```python
from build123d import *

# Parameters (mm, degrees)
SKETCH1_R           = 16.5
BOSS_EXTRUDE1_DEPTH = 82
SKETCH2_R           = 11
CUT_EXTRUDE1_DEPTH  = 276.268959383
SKETCH5_W           = 65
SKETCH5_H           = 35
CUT_EXTRUDE2_DEPTH  = 282.890049487
CUT_EXTRUDE3_DEPTH  = 40


with BuildPart() as part:
    # Sketch1 → Boss-Extrude1 (new body)
    with BuildSketch(Plane(origin=(0, 0, 0), x_dir=(1, 0, 0), z_dir=(0, 1, 0))):
        with BuildLine():
            Line((212.202700724, 100), (157.202700724, 100))
            ThreePointArc((157.202700724, 100), (151.120923095, 80.283600356), (134.9891913, 67.419244043))
            ThreePointArc((134.9891913, 67.419244043), (109.260251558, 61.670356138), (83, 64))
            Line((83, 64), (31.098692591, 64))
            Line((31.098692591, 64), (0, 35))
            Line((0, 35), (0, 0))
            Line((0, 0), (75.238209296, 0))
            ThreePointArc((75.238209296, 0), (96.859957606, -4.428268766), (115, -17))
            Line((115, -17), (157, -17))
            Line((157, -17), (176.293691384, 13.876360515))
            ThreePointArc((176.293691384, 13.876360515), (193.729138228, 30.421981775), (217, 36.440235832))
            Line((217, 36.440235832), (243, 36.440235832))
            Line((243, 36.440235832), (243, 80))
            Line((243, 80), (212.202700724, 100))
        make_face()
        with Locations(Location((135, 43, 0), (0, 0, 270))):
            Circle(SKETCH1_R, mode=Mode.SUBTRACT)
    extrude(amount=BOSS_EXTRUDE1_DEPTH)

    # Sketch2 → Cut-Extrude1 (cut, through all)
    with BuildSketch(Plane(origin=(0, 82, 0), x_dir=(1, 0, 0), z_dir=(0, 1, 0))):
        with Locations(Location((30, 35, 0), (0, 0, 270))):
            Circle(SKETCH2_R)
    extrude(amount=-CUT_EXTRUDE1_DEPTH, mode=Mode.SUBTRACT)

    # Sketch5 → Cut-Extrude2 (cut, through all)
    with BuildSketch(Plane(origin=(0, 0, -100), x_dir=(-1, 0, 0), z_dir=(0, 0, -1))):
        with Locations((-210.5, 64.5)):
            Rectangle(SKETCH5_W, SKETCH5_H)
    extrude(amount=-CUT_EXTRUDE2_DEPTH, mode=Mode.SUBTRACT)

    # Sketch6 → Cut-Extrude3 (cut)
    with BuildSketch(Plane(origin=(0, 15, 0), x_dir=(-1, 0, 0), z_dir=(0, -1, 0))):
        with BuildLine():
            Line((0, 12), (0, 35))
            Line((0, 35), (-31.098692591, 64))
            Line((-31.098692591, 64), (-74.689647512, 64))
            ThreePointArc((-74.689647512, 64), (-49.282519579, 20.85341744), (0, 12))
        make_face()
    extrude(amount=-CUT_EXTRUDE3_DEPTH, mode=Mode.SUBTRACT)


solid = part.part
```
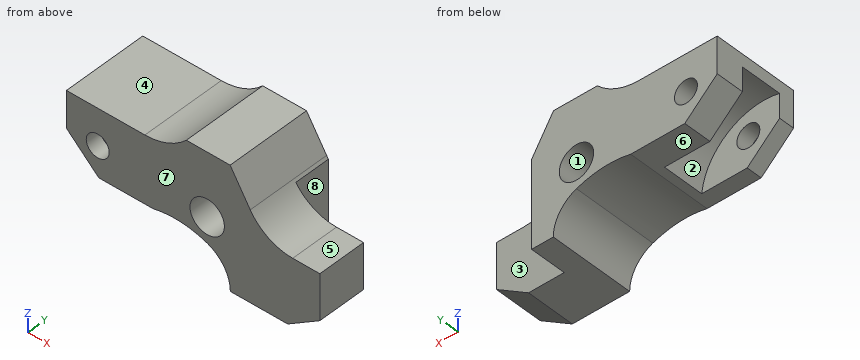
Geometry: final body of the model. Coordinates: model frame, mm. Face numbers are marked on the shaded views. A direction names the side the tool comes from. Round coordinates to 2 decimals unless told otherwise and drop trailing zeros. Loops run counter-clockwise (first coordinate to the right, second up) from the corner with the lowest first, then second, coordinate; pieces in that order, holes last.
Item 1: Mould query, pull axis Z, two halves, no side actions, for the marked faces 1, 2, 3 and 4. Classes: released by +Z, released by -Z, zero draft, split by the parting line, or undercut.
Checked values:
face 1: undercut
face 2: released by -Z
face 3: zero draft
face 4: released by +Z
Item 2: Section D-D, the plane x = 128. Output: boundary loops of the cut face in (y, z).
Checked values:
outline: (0, -65.02) - (82, -65.02) - (82, -57.94) - (0, -57.94) - close; (0, -28.06) - (82, -28.06) - (82, 17) - (0, 17) - close
Item 3: Reachability of the marked faces 5, 6, 7 and 8 from +Z, -Z, +X, -X, +Y, -Y: full face, straight path, thin tool, end or side. Return the list, or none.
Checked values:
face 5: +Z, +X, +Y, -Y
face 6: -Z, -X, +Y, -Y
face 7: +Z, -Z, +X, -X, -Y
face 8: +Z, -Z, +X, +Y
Item 4: Contact query for flat-ended pins moving along their axis: P1, Ø2, axis at x = 29, y = 33.5, coming from the +Z side; P2, Ø21, axis at x = 229.5, y = 14, coming from the +Z side; P3, Ø6, axis at y = 52, z = -83, coming from the +X side. Output: stop coordinate, or through.
Checked values:
P1: stops at z = 0
P2: stops at z = -36.44
P3: stops at x = 178
Item 5: Section A-A, the plane y = 67. Output: boundary loops of the cut face in (x, z).
Checked values:
outline: (0, -35) - (31.1, -64) - (83, -64) arc R85.85 cw to (134.99, -67.42) arc R35 cw to (157.2, -100) - (178, -100) - (178, -16.42) arc R48 cw to (176.29, -13.88) - (157, 17) - (115, 17) arc R55 cw to (75.24, 0) - (0, 0) - close; hole circle Ø22 at (30, -35); hole circle Ø33 at (135, -43)
Item 6: Section B-B, the plane z = -43. Output: boundary loops of the cut face in (x, y), plus the area to 3 significant figures.
Checked values:
outline: (8.58, 0) - (22.45, 0) - (22.45, 15) - (8.58, 15) - close; (8.58, 55) - (22.45, 55) - (22.45, 82) - (8.58, 82) - close; (37.55, 0) - (118.5, 0) - (118.5, 82) - (37.55, 82) - (37.55, 55) - (68.53, 55) - (68.53, 15) - (37.55, 15) - close; (151.5, 0) - (243, 0) - (243, 47) - (178, 47) - (178, 82) - (151.5, 82) - close
area: 11,200 mm2
Item 7: Section C-C, the plane y = 28.5. Output: boundary loops of the cut face in (x, z), plus the area to 3 significant figures.
Checked values:
outline: (0, -12) arc R60 cw to (74.69, -64) - (83, -64) arc R85.85 cw to (134.99, -67.42) arc R35 cw to (157.2, -100) - (212.2, -100) - (243, -80) - (243, -36.44) - (217, -36.44) arc R48 cw to (176.29, -13.88) - (157, 17) - (115, 17) arc R55 cw to (75.24, 0) - (0, 0) - close; hole circle Ø33 at (135, -43)
area: 13,200 mm2
Item 8: Line query: L1, parallel to X at y = 61, z = -43; L2, parallel to X at y = 65, z = -38; L3, parallel to Y at x = 208, z = -36.5. Output: solid intervals per line, ascending.
Checked values:
L1: x = 8.58 to 22.45, 37.55 to 118.5, 151.5 to 178
L2: x = 3.22 to 19.42, 40.58 to 119.28, 150.72 to 178
L3: y = 0 to 47
